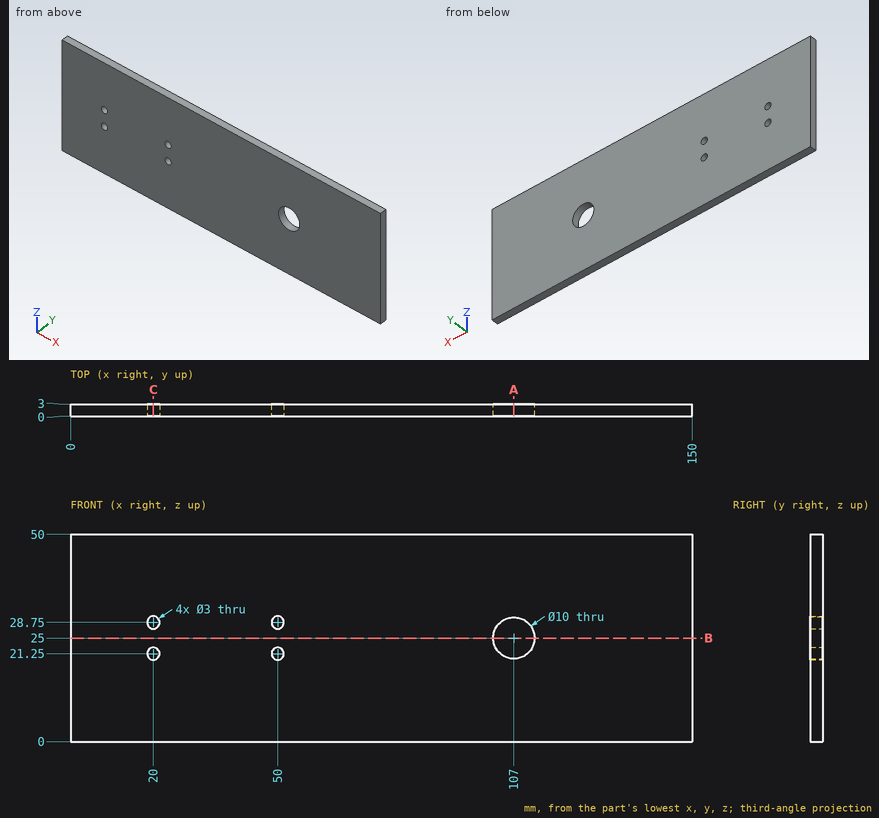
Can you work these out from the drawing? Everything is in mm from the part's minimum corner. Give positions to 0.01 mm unless a question says otherwise; leave off trailing zeros. Write each loop counter-clockwise with the first axis right and the second up, starting at its lowest first coordinate (ties: lowest second). Pieces come first, ordered by that corner, then holes. Notation, with made-up numbers: (24, 13.5) -> (50, 13.5) arc R15 cw to (50, 18.5) -> close; hole circle Ø1 at (68.25, 89). An arc over 180 degrees is marked (long way). Write each question's results on one line, items separated by ' | '.
Item 1: Suppose I cut it at A-A on x = 107. Write out the boundary of the cut face in (y, z), plus the area to 3 significant figures.
Output:
outline: (0, 0) -> (3, 0) -> (3, 20) -> (0, 20) -> close; (0, 30) -> (3, 30) -> (3, 50) -> (0, 50) -> close | area: 120 mm^2
Item 2: Suppose I cut it at B-B on z = 25. Write out the boundary of the cut face in (x, y), plus the area to 3 significant figures.
Output:
outline: (0, 0) -> (102, 0) -> (102, 3) -> (0, 3) -> close; (112, 0) -> (150, 0) -> (150, 3) -> (112, 3) -> close | area: 420 mm^2
Item 3: Suppose I cut it at C-C on x = 20. Write out the boundary of the cut face in (y, z).
Output:
outline: (0, 0) -> (3, 0) -> (3, 19.75) -> (0, 19.75) -> close; (0, 22.75) -> (3, 22.75) -> (3, 27.25) -> (0, 27.25) -> close; (0, 30.25) -> (3, 30.25) -> (3, 50) -> (0, 50) -> close
Item 4: For pin 1 Ø3.5 at (x, z) = (20, 28.75) entering from -Y, with a flat end and sliding along its axis, tell me the tip position at first contact or that it passes through.
Output:
pin 1: stops at y = 0
Item 5: If I drill on L1, parallel to X at y = 1.45, z = 21.25; L2, parallel to Z at x = 49, y = 1.8; L3, parallel to X at y = 2.25, z = 25.5, over which ranges is the centre line in solid material (lowest first)?
Output:
L1: x = 0 to 18.5, 21.5 to 48.5, 51.5 to 103.69, 110.31 to 150 | L2: z = 0 to 20.13, 22.37 to 27.63, 29.87 to 50 | L3: x = 0 to 102.03, 111.97 to 150
